Autodesk Inventor part; units mm, degrees
ref_plane "作業平面1" through (0, 6, 12) normal (0, 0, 1) x (1, 0, 0)
ref_plane "YZ Plane" through (0, 0, 0) normal (1, 0, 0) x (0, 1, 0)
ref_plane "XZ Plane" through (0, 0, 0) normal (0, 1, 0) x (-1, 0, 0)
sketch "スケッチ1" plane through (0, 0, 0) normal (0, 1, 0) x (-1, 0, 0)
  circle A0 centre (0, 0) radius 28.5
  line L0 (-28.5, 0) -> (28.5, 0) construction
  circle A1 centre (23.5, 0) radius 2.5
  circle A2 centre (11.75, 20.3516) radius 2.5
  circle A3 centre (-11.75, 20.3516) radius 2.5
  circle A4 centre (-23.5, 0) radius 2.5
  circle A5 centre (-11.75, -20.3516) radius 2.5
  circle A6 centre (11.75, -20.3516) radius 2.5
  circle A7 centre (0, 0) radius 6
  dimension "d0" = 57
  dimension "d1" = 5
  dimension "d2" = 23.5
  dimension "d6" = 360
  dimension "d10" = 12
extrude "押し出し1" add sketch "スケッチ1" along normal blind 6
sketch "スケッチ2" plane through (0, 6, 0) normal (0, 1, 0) x (1, 0, 0)
  circle A0 centre (0, 0) radius 12
  circle A1 centre (0, 0) radius 6
  dimension "d11" = 24
extrude "押し出し2" add sketch "スケッチ2" along normal blind 20
ref_plane "作業平面1" through (0, 6, 12) normal (0, 0, 1) x (1, 0, 0)
sketch "スケッチ3" plane through (0, 6, 12) normal (0, 0, 1) x (1, 0, 0)
  line L0 (12, 20) -> (-12, 20)
  line L1 (12, 20) -> (-12, 20)
  line L2 (-12, 0) -> (12, 0)
  circle A0 centre (0, 10) radius 2.5
  line L3 (0, 0) -> (0, 20) construction
  point P0 (0, -6)
  dimension "d14" = 20
  dimension "d15" = 5
  dimension "d16" = 10
extrude "押し出し3" cut sketch "スケッチ3" against normal up to surface
thread "ねじ1"
equation "\"d16\" = 0.5 * d14"
properties part number "frange" material "ステンレス鋼"
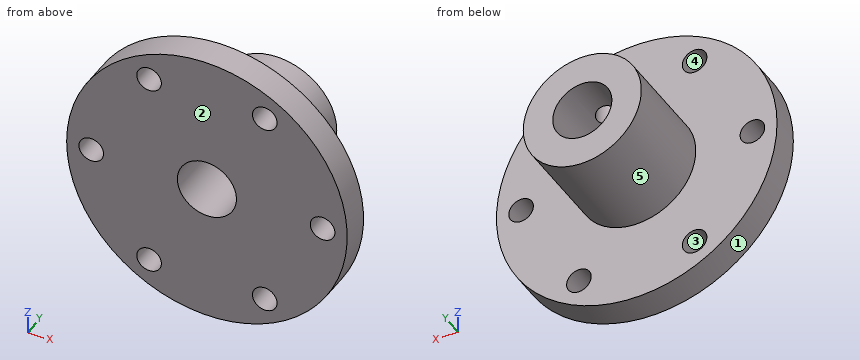
Read the model definition and answer for the solid it produces. Units are mm, in the model's axes. Face numbers are marked on the shaded views. A direction names the side the tool comes from. Round coordinates to 2 decimals unless told otherwise and drop trailing zeros. Write each loop counter-clockwise with the first axis right and the second up, starting at its lowest first coordinate (ties: lowest second). Pieces come first, ordered by that corner, then holes. Notation, with made-up numbers: (38, 40) - (81, 40) arc R15 cw to (81, 45) - close; hole circle Ø8 at (-0.5, 81). An arc over 180 degrees is marked (long way). One line per question, with ' | ' between items. Start each with the question number.
1. Section A-A (x = -23) is taken. Determine the outline of the cut face in (y, z).
2. Section C-C (z = 19) is taken. Determine the outline of the cut face in (x, y), and give its area (3 significant figures).
3. Each of these flat-tipped pins is pushed along its axis until it touches: pin 1 (1.5 mm diameter, centred on y = 5.5, z = 15, fed in from -X); pin 2 (3 mm diameter, centred on y = 8, z = -7, fed in from -X); pin 3 (4.5 mm diameter, centred on x = 11.75, z = -20.35, fed in from +Y); pin 4 (5 mm diameter, centred on x = 12.5, y = 8, fed in from -Z). Where does it stop, or does it pass through?
4. Section B-B (y = 8.75) is taken. Determine the outline of the cut face in (x, z), and give its area (3 significant figures).
5. For a pull along Z with two mould halves and no side action, classify the marked faces 1, 2 and 3 as +Z half, -Z half, draft (parallel to the pull), parting line (faces both ways), or undercut.
6. Find the intervals of material crossed by probe 1 along Z at (x, y) = (-13, 4.25); probe 2 along Z at (x, y) = (-11.75, 1.75); probe 3 along Y at (x, z) = (0, 10.75), in increasing order. Write a range as [from, to].
7. For the marked faces 4 and 5, determine the directions among +Z, -Z, +X, -X, +Y, -Y from which every point of the face is accessible in a straight line to the end or side of a thin tool.
Filled in:
1) outline: (0, -16.83) - (6, -16.83) - (6, -2.45) - (0, -2.45) - close; (0, 2.45) - (6, 2.45) - (6, 16.83) - (0, 16.83) - close
2) outline: (-21.24, 0) - (-13.85, 0) - (-13.85, 6) - (-21.24, 6) - close; (-9.65, 0) - (9.65, 0) - (9.65, 6) - (-9.65, 6) - close; (13.85, 0) - (21.24, 0) - (21.24, 6) - (13.85, 6) - close | area: 204 mm²
3) pin 1: x = -24.68 | pin 2: x = -10.67 | pin 3: through | pin 4: z = -26.29
4) outline: circle Ø24 at (0, 0); hole circle Ø12 at (0, 0) | area: 339 mm²
5) face 1: parting line | face 2: draft | face 3: undercut
6) probe 1: [-25.36, -22.52], [-18.19, 18.19], [22.52, 25.36] | probe 2: [-25.97, -22.85], [-17.85, 17.85], [22.85, 25.97] | probe 3: [0, 13.5], [18.5, 26]
7) face 4: +Y, -Y | face 5: +Y
